Source: three-view drawing plus pictorial views. Frame: mm from the lowest corner of the part. Give positions to 0.01 mm unless a question says otherwise; leave off trailing zeros. Loops run counter-clockwise (first coordinate to the right, second up) from the corner with the lowest first, then second, coordinate; pieces in that order, holes last.
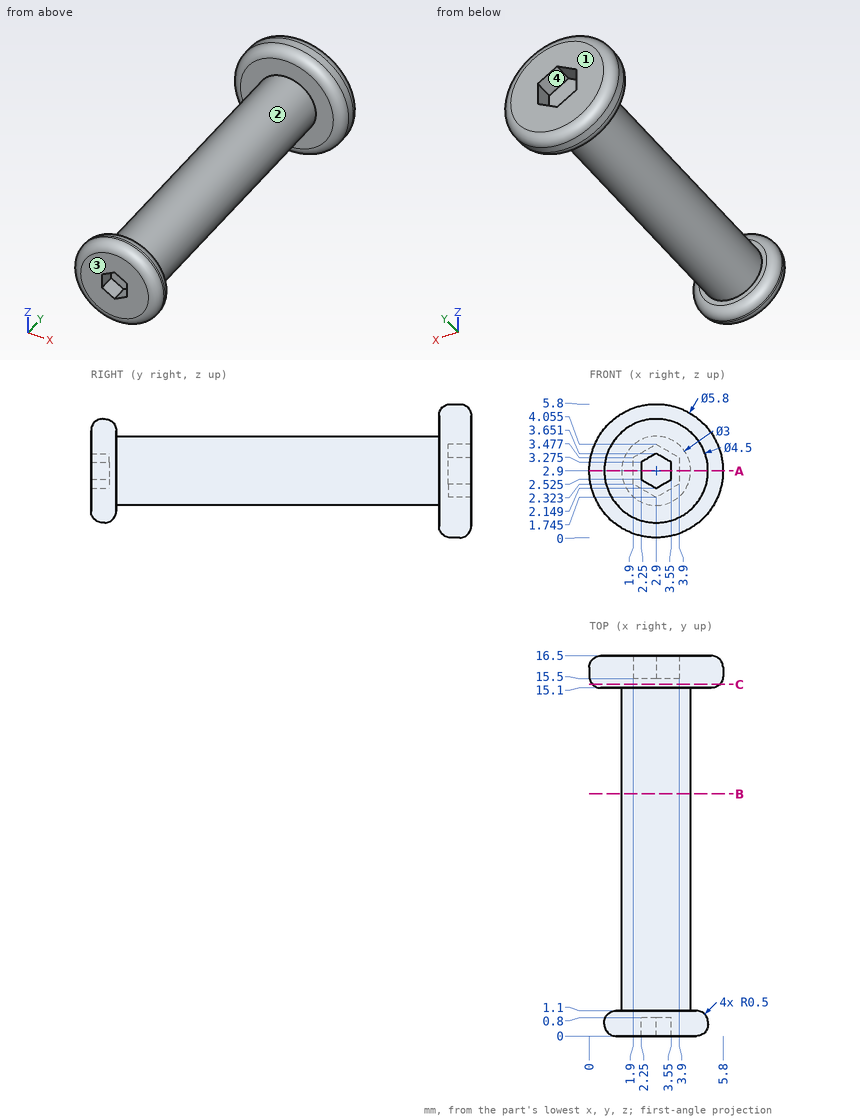
(1) Cut plane C-C (y = 15.25). Return the cut outline in (x, z) (1 decimal), and give its area (3 significant figures).
Values follow:
outline: circle Ø5.5 at (2.9, 2.9)
area: 23.9 mm2
(2) Cut plane B-B (y = 10.5). Return the cut outline in (x, z).
Values follow:
outline: circle Ø3 at (2.9, 2.9)
(3) Cut plane A-A (z = 2.9). Return the cut outline in (x, y), and give its area (3 significant figures).
Values follow:
outline: (0, 15.6) arc R0.5 ccw to (0.5, 15.1) - (1.4, 15.1) - (1.4, 1.1) - (1.15, 1.1) arc R0.5 ccw to (0.65, 0.6) - (0.65, 0.5) arc R0.5 ccw to (1.15, 0) - (2.25, 0) - (2.25, 0.8) - (3.55, 0.8) - (3.55, 0) - (4.65, 0) arc R0.5 ccw to (5.15, 0.5) - (5.15, 0.6) arc R0.5 ccw to (4.65, 1.1) - (4.4, 1.1) - (4.4, 15.1) - (5.3, 15.1) arc R0.5 ccw to (5.8, 15.6) - (5.8, 16) arc R0.5 ccw to (5.3, 16.5) - (3.9, 16.5) - (3.9, 15.5) - (1.9, 15.5) - (1.9, 16.5) - (0.5, 16.5) arc R0.5 ccw to (0, 16) - close
area: 51.6 mm2
(4) Mould query, pull axis Y, two halves, no side actions, for the marked faces 1, 2, 3 and 4. Classes: +Y half, -Y half, draft (parallel to the pull), parting line (faces both ways), or undercut.
Values follow:
face 1: +Y half
face 2: undercut
face 3: -Y half
face 4: draft
(5) Pin query (flat end, axial travel): pin 1 Ø1 at (x, z) = (3, 2.5) entering from +Y; pin 2 Ø0.8 at (y, z) = (0, 3) entering from -X; pin 3 Ø1 at (y, z) = (6.5, 2) entering from +X (1 decimal). Return the tip coordinate at first contact, or that it passes through.
Values follow:
pin 1: stops at y = 15.5
pin 2: stops at x = 0.66
pin 3: stops at x = 4.3
(6) Ray query, probe 1 along Y at (x, z) = (2.2, 4.35); probe 2 along Y at (x, z) = (5.1, 3.9); probe 3 along X at (y, z) = (3.25, 2.85). Return the intervals inside material, ascending.
Values follow:
probe 1: y = 0 to 1.1, 15.1 to 16.5
probe 2: y = 15.1 to 16.5
probe 3: x = 1.4 to 4.4
